```python
from build123d import *

# Parameters (mm, degrees)
BOSS_EXTRUDE1_DEPTH      = 22
BOSS_EXTRUDE1_DEPTH_BACK = 22
SKETCH2_W                = 38
SKETCH2_H                = 20
CUT_EXTRUDE1_DEPTH       = 105.423416914
SKETCH3_W                = 7
SKETCH3_H                = 44
BOSS_EXTRUDE2_DEPTH      = 36
SKETCH5_W                = 34
SKETCH5_H                = 50
CUT_EXTRUDE3_DEPTH       = 109.047443283
SKETCH6_W                = 20.5
SKETCH6_H                = 54.25
CUT_EXTRUDE4_DEPTH       = 111.605436123
SKETCH20_W               = 28.5
SKETCH20_H               = 34
SKETCH20_R               = 1.7
SKETCH20_R_2             = 5
BOSS_EXTRUDE5_DEPTH      = 4
SKETCH21_W               = 3
SKETCH21_H               = 36
CUT_EXTRUDE12_DEPTH      = 66.777085676
SKETCH22_W               = 4
SKETCH22_H               = 25
CUT_EXTRUDE14_DEPTH      = 66.054784605


with BuildPart() as part:
    # Sketch1 → Boss-Extrude1 (new, two sides: drawn at the far end of the back side and taken through both)
    with BuildSketch(Plane.XY.offset(-BOSS_EXTRUDE1_DEPTH_BACK)):
        with BuildLine():
            Line((10.25, -60), (10.25, 0))
            ThreePointArc((10.25, 0), (0, -10.25), (-10.25, 0))
            Line((-10.25, 0), (-10.25, -60))
            Line((-10.25, -60), (-10.25, -100))
            Line((-10.25, -100), (10.25, -100))
            Line((10.25, -100), (10.25, -60))
        make_face()
        with BuildLine():
            Line((10.25, 0), (9.2, 0))
            ThreePointArc((9.2, 0), (8.816088231, -0.879772698), (7.91, -1.196620241))
            ThreePointArc((7.91, -1.196620241), (5.656854249, -5.656854249), (1.196620241, -7.91))
            ThreePointArc((1.196620241, -7.91), (1.199154762, -7.954968281), (1.2, -8))
            ThreePointArc((1.2, -8), (-0.045031719, -9.199154762), (-1.196620241, -7.91))
            ThreePointArc((-1.196620241, -7.91), (-5.656854249, -5.656854249), (-7.91, -1.196620241))
            ThreePointArc((-7.91, -1.196620241), (-8.816088231, -0.879772698), (-9.2, 0))
            Line((-9.2, 0), (-10.25, 0))
            ThreePointArc((-10.25, 0), (0, -10.25), (10.25, 0))
        make_face()
        with BuildLine():
            ThreePointArc((7.91, -1.196620241), (7.120227302, -0.816088231), (6.8, 0))
            Line((6.8, 0), (4.2, 0))
            ThreePointArc((4.2, 0), (0, -4.2), (-4.2, 0))
            Line((-4.2, 0), (-6.8, 0))
            ThreePointArc((-6.8, 0), (-7.120227302, -0.816088231), (-7.91, -1.196620241))
            ThreePointArc((-7.91, -1.196620241), (-5.656854249, -5.656854249), (-1.196620241, -7.91))
            ThreePointArc((-1.196620241, -7.91), (0, -6.8), (1.196620241, -7.91))
            ThreePointArc((1.196620241, -7.91), (5.656854249, -5.656854249), (7.91, -1.196620241))
        make_face()
        with BuildLine():
            Line((4.2, 0), (6.8, 0))
            ThreePointArc((6.8, 0), (7.120227302, 0.816088231), (7.91, 1.196620241))
            ThreePointArc((7.91, 1.196620241), (5.656854249, 5.656854249), (1.196620241, 7.91))
            ThreePointArc((1.196620241, 7.91), (0, 6.8), (-1.196620241, 7.91))
            ThreePointArc((-1.196620241, 7.91), (-5.656854249, 5.656854249), (-7.91, 1.196620241))
            ThreePointArc((-7.91, 1.196620241), (-7.120227302, 0.816088231), (-6.8, 0))
            Line((-6.8, 0), (-4.2, 0))
            ThreePointArc((-4.2, 0), (0, 4.2), (4.2, 0))
        make_face()
        with BuildLine():
            ThreePointArc((7.91, 1.196620241), (8.816088231, 0.879772698), (9.2, 0))
            Line((9.2, 0), (10.25, 0))
            ThreePointArc((10.25, 0), (0, 10.25), (-10.25, 0))
            Line((-10.25, 0), (-9.2, 0))
            ThreePointArc((-9.2, 0), (-8.816088231, 0.879772698), (-7.91, 1.196620241))
            ThreePointArc((-7.91, 1.196620241), (-5.656854249, 5.656854249), (-1.196620241, 7.91))
            ThreePointArc((-1.196620241, 7.91), (-0.045031719, 9.199154762), (1.2, 8))
            ThreePointArc((1.2, 8), (1.199154762, 7.954968281), (1.196620241, 7.91))
            ThreePointArc((1.196620241, 7.91), (5.656854249, 5.656854249), (7.91, 1.196620241))
        make_face()
    extrude(amount=BOSS_EXTRUDE1_DEPTH + BOSS_EXTRUDE1_DEPTH_BACK)

    # Sketch2 → Cut-Extrude1 (cut, through all)
    with BuildSketch(Plane.ZY.offset(10.25)):
        with Locations((0, 0.25)):
            Rectangle(SKETCH2_W, SKETCH2_H)
    extrude(amount=-CUT_EXTRUDE1_DEPTH, mode=Mode.SUBTRACT)

    # Sketch3 → Boss-Extrude2 (add)
    with BuildSketch(Plane(origin=(0, -9.75, 0), x_dir=(1, 0, 0), z_dir=(0, 1, 0))):
        with Locations((-13.75, 0)):
            Rectangle(SKETCH3_W, SKETCH3_H)
        with Locations((13.75, 0)):
            Rectangle(SKETCH3_W, SKETCH3_H)
    extrude(amount=-BOSS_EXTRUDE2_DEPTH)

    # Sketch5 → Cut-Extrude3 (cut, through all)
    with BuildSketch(Plane.ZY.offset(17.25)):
        with Locations((0, -34.75)):
            Rectangle(SKETCH5_W, SKETCH5_H)
    extrude(amount=-CUT_EXTRUDE3_DEPTH, mode=Mode.SUBTRACT)

    # Sketch6 → Cut-Extrude4 (cut, through all)
    with BuildSketch(Plane.XY.offset(22)):
        with Locations((0, -72.875)):
            Rectangle(SKETCH6_W, SKETCH6_H)
    extrude(amount=-CUT_EXTRUDE4_DEPTH, mode=Mode.SUBTRACT)


with BuildPart() as cut_extrude4_piece_1:
    # of the separate pieces the step leaves, piece 1, a body of its own (cut_extrude4_pieces)
    add(part.part.solids().sort_by_distance((10.25, 0, -22))[0])



with BuildPart() as cut_extrude4_piece_2:
    # of the separate pieces the step leaves, piece 2, a body of its own (cut_extrude4_pieces)
    add(part.part.solids().sort_by_distance((17.25, -45.75, 22))[0])


with BuildPart() as cut_extrude4_piece_1_1:
    add(cut_extrude4_piece_1.part)

    add(cut_extrude4_piece_2.part)  # Boss-Extrude5 merges Cut-Extrude4 piece 2
    # Sketch20 → Boss-Extrude5 (add)
    with BuildSketch(Plane.XZ.offset(45.75)):
        Rectangle(SKETCH20_W, SKETCH20_H)
        with Locations(Location((-8.25, -9, 0), (0, 0, 270))):
            Circle(SKETCH20_R, mode=Mode.SUBTRACT)
        with Locations(Location((8.25, -9, 0), (0, 0, 270))):
            Circle(SKETCH20_R, mode=Mode.SUBTRACT)
        with Locations(Location((-8.25, 9, 0), (0, 0, 270))):
            Circle(SKETCH20_R, mode=Mode.SUBTRACT)
        with Locations(Location((0, 0, 0), (0, 0, 270))):
            Circle(SKETCH20_R_2, mode=Mode.SUBTRACT)
        with Locations(Location((8.25, 9, 0), (0, 0, 270))):
            Circle(SKETCH20_R, mode=Mode.SUBTRACT)
    extrude(amount=-BOSS_EXTRUDE5_DEPTH)

    # Sketch21 → Cut-Extrude12 (cut, through all)
    with BuildSketch(Plane(origin=(0, 0, -22), x_dir=(-1, 0, 0), z_dir=(0, 0, -1))):
        with Locations((-15.75, -27.75)):
            Rectangle(SKETCH21_W, SKETCH21_H)
        with Locations((15.75, -27.75)):
            Rectangle(SKETCH21_W, SKETCH21_H)
    extrude(amount=-CUT_EXTRUDE12_DEPTH, mode=Mode.SUBTRACT)

    # Sketch22 → Cut-Extrude14 (cut, through all)
    with BuildSketch(Plane(origin=(0, 0, -22), x_dir=(-1, 0, 0), z_dir=(0, 0, -1))):
        with Locations((12.25, -22.25)):
            Rectangle(SKETCH22_W, SKETCH22_H)
    extrude(amount=-CUT_EXTRUDE14_DEPTH, mode=Mode.SUBTRACT)


solid = cut_extrude4_piece_1_1.part
```
Can you work these out from the model? Positions are in its coordinate system, mm. A direction names the side the tool comes from. Give positions to 0.01 mm unless a question says otherwise; leave off trailing zeros. Order: outer loops, then holes, each group sorted by start corner. A loop starts at its lowest first (then second) coordinate and runs counter-clockwise, first axis right, second up. Notation, with made-up numbers: M 71.5,51.25 L 99.5,51.25 A11 cw 99.5,69.25 Z; hole C -10,-36.5 d5. An arc over 180 degrees is marked long. Write item = value, one per line. Start each with the question number.
Q1. We'd pull the mould along Z, two halves only. Please class faces 1 (the flat face through (2, -9.75, -18)), 2 (the flat face through (0, -24, 22)), 3 (the flat face through (10.25, -5, -21)): pulls with the +Z half, pulls with the -Z half, needs draft (parallel to the pull), parting line crosses it, or undercut.
Q2. I need wall thicknesses on probe 1 along X at (y, z) = (-42, 9); probe 2 along Z at (x, y) = (-7.75, -22); probe 3 along Z at (x, y) = (-6.25, 8). Which ranges of each line are inside material? Lowest first, please. Write a range as [from, to].
Q3. Suppose I cut it at A-A (z = -3). Write out the boundary of the cut face in (x, y), plus the area to 3 significant figures.
Q4. Will these pins go through, and if not, where does the flat tip stop? pin 1 Ø2.5 at (x, z) = (5.5, -19.5) entering from +Y; pin 2 Ø2 at (x, z) = (-11.5, -19.5) entering from +Y; pin 3 Ø2 at (x, z) = (-6, -6) entering from +Y.
Q5. Suppose I cut it at D-D (z = 9). Write out the boundary of the cut face in (x, y), plus the area to 3 significant figures.
Q6. Suppose I cut it at C-C (x = 0). Count the separate pieces of the cut face and the enclosed holes in it, plus the area to 3 significant figures.
Q7. Suppose I cut it at B-B (y = -11.5). Write out the boundary of the cut face in (x, z), plus the area to 3 significant figures.
Q8. For faces 4 (the flat face through (2, -9.75, 18)), 5 (the flat face through (2, -4, -19)), 6 (the flat face through (10.25, -5, 20)), 7 (the flat face through (-12, -34.75, -20)), which set-ups out of +Z, -Z, +X, -X, +Y, -Y let a thin tool reach every point of the face, with its end or its side?
Check result:
q1.face_1 = undercut
q1.face_2 = pulls with the +Z half
q1.face_3 = needs draft
q2.probe_1 = [-14.25, -9.95], [-6.55, 6.55], [9.95, 14.25]
q2.probe_2 = [-22, -17], [17, 22]
q2.probe_3 = [-22, -19], [19, 22]
q3.outline = M -14.25,-45.75 L -4,-45.75 L -4,-41.75 L -14.25,-41.75 Z; M 4,-45.75 L 14.25,-45.75 L 14.25,-41.75 L 4,-41.75 Z
q3.area = 82.0 mm2
q4.pin_1 = 9.33
q4.pin_2 = -34.75
q4.pin_3 = -41.75
q5.outline = M -14.25,-45.75 L -9.95,-45.75 L -9.95,-41.75 L -14.25,-41.75 Z; M -6.55,-45.75 L 6.55,-45.75 L 6.55,-41.75 L -6.55,-41.75 Z; M 9.95,-45.75 L 14.25,-45.75 L 14.25,-41.75 L 9.95,-41.75 Z
q5.area = 86.8 mm2
q6.separate_pieces = 8
q6.enclosed_holes = 0
q6.area = 497 mm2
q7.outline = M -10.25,-22 L 14.25,-22 L 14.25,-17 L -10.25,-17 Z; M -10.25,17 L 14.25,17 L 14.25,22 L -10.25,22 Z
q7.area = 245 mm2
q8.face_4 = +X, +Y
q8.face_5 = +X, -X, +Y
q8.face_6 = +Z, -Z, +X, +Y
q8.face_7 = +Z, -Z, -X, +Y
